The figure shows three views and two pictorial views of one solid part (mm, origin at its lowest corner). Answer the questions. A direction names the side the tool comes from. Coordinates: 2 decimals unless noted, no trailing zeros. Order: outer loops, then holes, each group sorted by start corner. A loop starts at its lowest first (then second) coordinate and runs counter-clockwise, first axis right, second up.
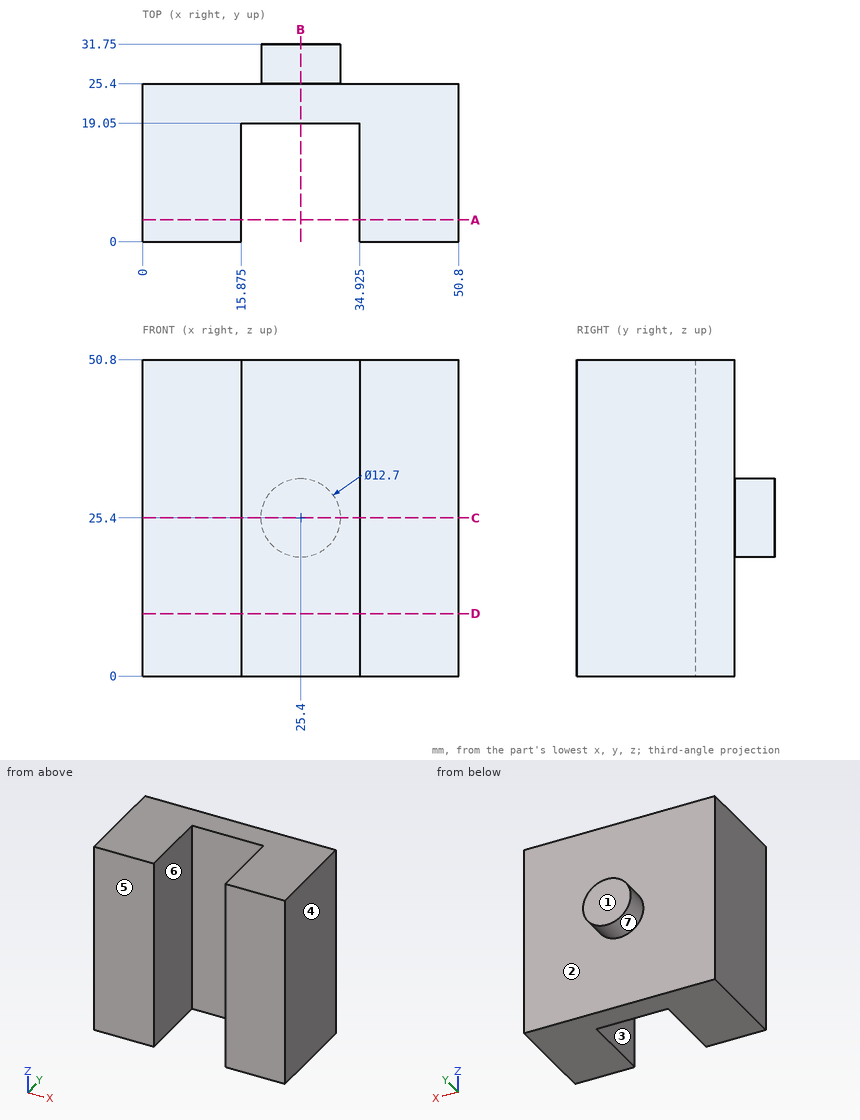
1) A cutting plane is placed at B-B, the plane x = 25.4. Write down the section's boundary in (y, z).
2) A cutting plane is placed at A-A, the plane y = 3.5. Write down the section's boundary in (x, z) (3 decimals), plus the area to 3 significant figures.
3) For the marked faces 1, 2 and 3, determine the directions among +Z, -Z, +X, -X, +Y, -Y from which every point of the face is accessible in a straight line to the end or side of a thin tool.
4) Each of these flat-tipped pins is pushed along its axis until it touches: P1, Ø1, axis at y = 14, z = 37, coming from the -X side; P2, Ø6, axis at x = 9.5, z = 25, coming from the +Y side. Where does it stop, or does it pass through?
5) A cutting plane is placed at C-C, the plane z = 25.4. Write down the section's boundary in (x, y) (3 decimals).
6) The mould has two halves that part along X. Classify the marked faces 4, 5, 6 and 7: released by +X, released by -X, zero draft, split by the parting line, or undercut.
7) A cutting plane is placed at D-D, the plane z = 10. Write down the section's boundary in (x, y) (3 decimals), plus the area to 3 significant figures.
8) Straight lines are drawn through the part: probe 1 along X at (y, z) = (3.5, 45) (3 decimals); probe 2 along Y at (x, z) = (3, 36); probe 3 along Y at (x, z) = (25, 16). For each, find the intervals that lie inside material, in ascending order.
Working result:
1. outline: (19.05, 0) - (25.4, 0) - (25.4, 19.05) - (31.75, 19.05) - (31.75, 31.75) - (25.4, 31.75) - (25.4, 50.8) - (19.05, 50.8) - close
2. outline: (0, 0) - (15.875, 0) - (15.875, 50.8) - (0, 50.8) - close; (34.925, 0) - (50.8, 0) - (50.8, 50.8) - (34.925, 50.8) - close
2. area: 1,610 mm2
3. face 1: +Z, -Z, +X, -X, +Y
3. face 2: +Y
3. face 3: +Z, -Z, -Y
4. P1: stops at x = 0
4. P2: stops at y = 25.4
5. outline: (0, 0) - (15.875, 0) - (15.875, 19.05) - (34.925, 19.05) - (34.925, 0) - (50.8, 0) - (50.8, 25.4) - (31.75, 25.4) - (31.75, 31.75) - (19.05, 31.75) - (19.05, 25.4) - (0, 25.4) - close
6. face 4: released by +X
6. face 5: zero draft
6. face 6: undercut
6. face 7: split by the parting line
7. outline: (0, 0) - (15.875, 0) - (15.875, 19.05) - (34.925, 19.05) - (34.925, 0) - (50.8, 0) - (50.8, 25.4) - (0, 25.4) - close
7. area: 927 mm2
8. probe 1: x = 0 to 15.875, 34.925 to 50.8
8. probe 2: y = 0 to 25.4
8. probe 3: y = 19.05 to 25.4
